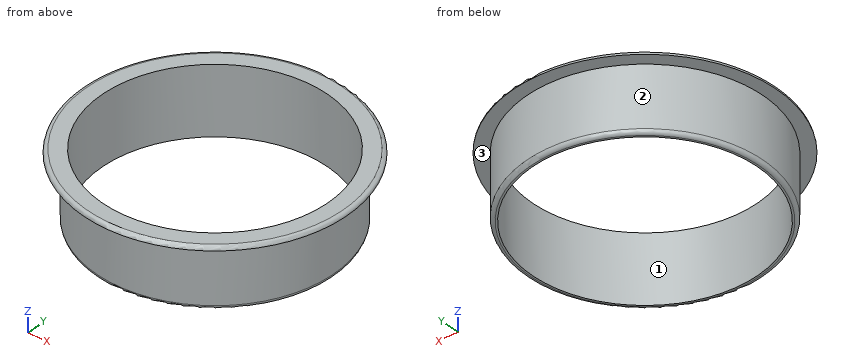
Autodesk Inventor part; units mm, degrees
ref_plane "YZ Plane" through (0, 0, 0) normal (1, 0, 0) x (0, 1, 0)
ref_plane "XZ Plane" through (0, 0, 0) normal (0, 1, 0) x (-1, 0, 0)
ref_plane "XY Plane" through (0, 0, 0) normal (0, 0, 1) x (1, 0, 0)
sketch "Sketch1" plane through (0, 0, 0) normal (0, 0, 1) x (1, 0, 0)
  circle A0 centre (0, 0) radius 31.5
  circle A1 centre (0, 0) radius 30
  circle A2 centre (0, 0) radius 35
  dimension "d0" = 63
  dimension "d1" = 60
  dimension "d2" = 70
extrude "Extrusion1" add sketch "Sketch1" along normal blind 1 contours A0 | A2
extrude "Extrusion2" add sketch "Sketch1" against normal blind 17 contours A0
fillet "Fillet1" radius 1 1 edges at (-35, 0, 1)
fillet "Fillet2" radius 1 1 edges at (-31.5, 0, -17)
properties part number "Hole64mm"
The listing builds one solid part. Answer for the finished solid, in the listing's coordinates (mm). Face numbers are marked on the shaded views. Coordinates: 2 decimals unless noted, no trailing zeros. Loops run counter-clockwise (first coordinate to the right, second up) from the corner with the lowest first, then second, coordinate; pieces in that order, holes last. Notation, with made-up numbers: M 82.25,59 L 133.25,59 A17 cw 133.25,79 Z; hole C -29.5,15 d1. An arc over 180 degrees is marked long. Answer as a JSON object with one key per item and string values. Group by question number.
Item 1: Consider L1, parallel to Y at x = 0, z = -4; L2, parallel to Y at x = 3, z = -11.75; L3, parallel to X at y = 7.5, z = -7.5. Determine where each line is inside the solid, lowest interval first.
Item 2: Section C-C (z = -10.75) is taken. Write down the section's boundary in (x, y), and give its area (3 significant figures).
Item 3: Each of these flat-tipped pins is pushed along its axis until it touches: P1, Ø8, axis at y = 18, z = -7.5, coming from the -X side; P2, Ø10, axis at y = -5.5, z = -2, coming from the -X side; P3, Ø1.5, axis at y = 17.5, z = -1, coming from the -X side. Where does it stop, or does it pass through?
Item 4: Determine the mould class of the marked faces 1, 2 and 3 for opening direction X: +X half, -X half, draft (parallel to the pull), parting line (faces both ways), or undercut.
Solved:
{
 "1": {"L1": "y = -31.5 to -30, 30 to 31.5", "L2": "y = -31.36 to -29.85, 29.85 to 31.36", "L3": "x = -30.59 to -29.05, 29.05 to 30.59"},
 "2": {"outline": "C 0,0 d63; hole C 0,0 d60", "area": "290 mm2"},
 "3": {"P1": "stops at x = -28.22", "P2": "stops at x = -34.99", "P3": "stops at x = -26.68"},
 "4": {"face 1": "undercut", "face 2": "parting line", "face 3": "draft"}
}
